from build123d import *


with BuildPart() as part:
    # Sketch → AdditiveLoft section 0
    with BuildSketch(Plane.XY):
        Polygon((-50, 0), (-65.332946, 31.462689), (-31.17449, 39.091574), (-16.135905, 70.696019), (11.126047, 48.746396), (45.211801, 56.693806), (45.048443, 21.694187), (72.514099, 0), (45.048443, -21.694187), (45.211801, -56.693806), (11.126047, -48.746396), (-16.135905, -70.696019), (-31.17449, -39.091574), (-65.332946, -31.462689), align=None)
    # Sketch001 → AdditiveLoft section 1
    with BuildSketch(Plane.XY.offset(120)):
        Polygon((-45.048443, 21.694187), (-45.211801, 56.693806), (-11.126047, 48.746396), (16.135905, 70.696019), (31.17449, 39.091574), (65.332946, 31.462689), (50, 0), (65.332946, -31.462689), (31.17449, -39.091574), (16.135905, -70.696019), (-11.126047, -48.746396), (-45.211801, -56.693806), (-45.048443, -21.694187), (-72.514099, 0), align=None)
    loft()


solid = part.part
Verification items for the finished model (mm, model axes). Round coordinates to 2 decimals unless told otherwise and drop trailing zeros. Use a Markdown table: item, result. Add a question column.
1. Section check A-A, the plane x = 61.5. Give the number of separate pieces and of enclosed holes in the cut face, plus the area to 3 significant figures.
2. Gauge pin test, flat ends, axial feed: pin 1 (10 mm diameter, centred on y = -38, z = 42.5, fed in from -X); pin 2 (8 mm diameter, centred on x = -5, z = 24, fed in from +Y); pin 3 (5 mm diameter, centred on x = 52, z = 46.5, fed in from +Y). Record the tip position at first contact, or that the pin passes through.
3. Thickness scan on probe 1 along X at (y, z) = (-14.5, 75); probe 2 along Y at (x, z) = (-16, 41.5); probe 3 along Y at (x, z) = (10, 64.5). Record the ranges inside material, lowest first. Write a range as [from, to].
Checks:
| question | item | result |
|---|---|---|
| 1 | separate pieces | 3 |
| 1 | enclosed holes | 0 |
| 1 | area | 1,050 mm^2 |
| 2 | pin 1 | stops at x = -51.82 |
| 2 | pin 2 | stops at y = 63.37 |
| 2 | pin 3 | stops at y = 31.84 |
| 3 | probe 1 | x = [-57.54, 58.07] |
| 3 | probe 2 | y = [-61.78, 61.78] |
| 3 | probe 3 | y = [-60.31, 60.31] |
